Design review of the part shown in the three views and the two pictorial views. Dimensions are in mm from the part's minimum x, y and z. Give positions to 0.01 mm unless a question says otherwise; leave off trailing zeros. Loops run counter-clockwise (first coordinate to the right, second up) from the corner with the lowest first, then second, coordinate; pieces in that order, holes last.
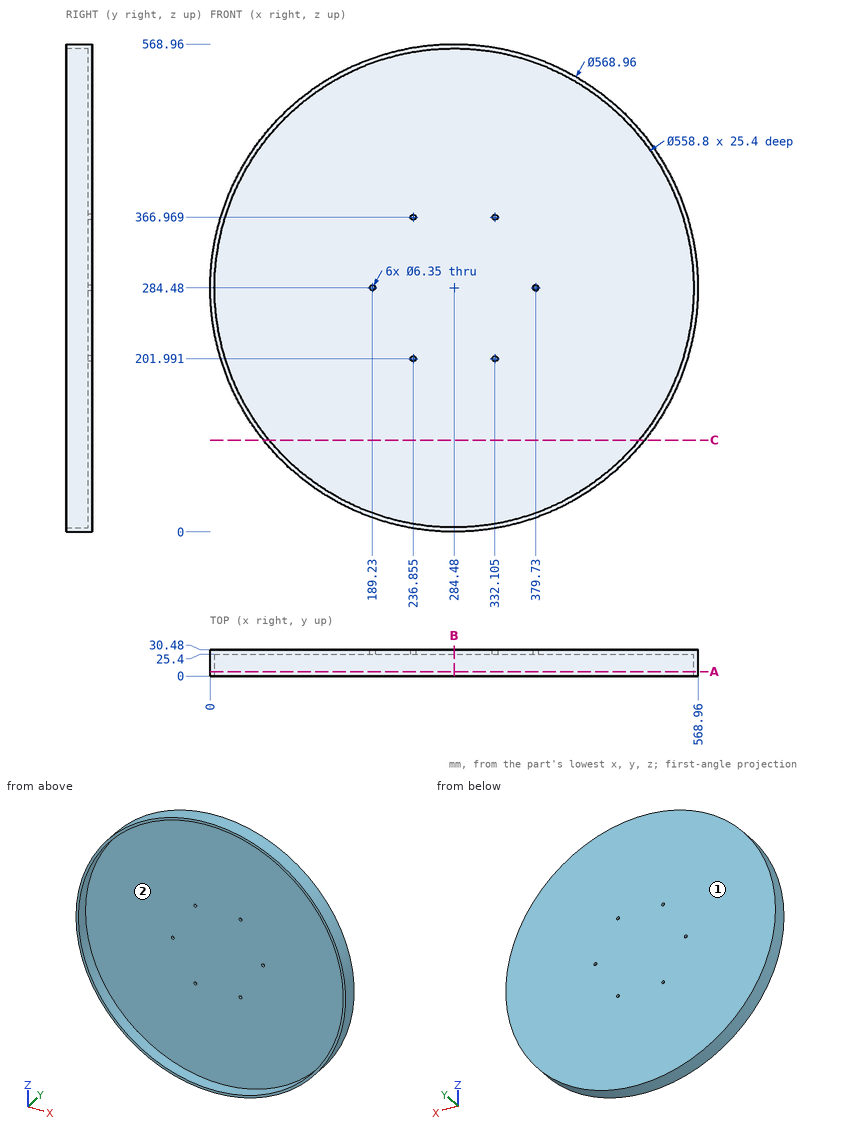
Q1. Mouldability with a two-part tool opening along X and no side actions: class the marked faces 1 and 2 as +X half, -X half, draft (parallel to the pull), parting line (faces both ways), or undercut.
Answers:
face 1: draft
face 2: undercut
Q2. For probe 1 along Z at (x, y) = (284, 12); probe 2 along Y at (x, z) = (367, 379); probe 3 along Z at (x, y) = (189.23, 27.1) (1 decimal), list the stretches that pass through material, from the lowest coordinate up.
Answers:
probe 1: z = 0 to 5.08, 563.88 to 568.96
probe 2: y = 25.4 to 30.48
probe 3: z = 16.4 to 281.3, 287.7 to 552.5
Q3. Consider section A-A on y = 5. Give the boundary of the cut face in (x, z), plus the area to 3 significant figures.
Answers:
outline: circle Ø568.96 at (284.48, 284.48); hole circle Ø558.8 at (284.48, 284.48)
area: 9,000 mm2
Q4. For pin 1 Ø5.5 at (x, z) = (236.86, 201.99) entering from -Y; pin 2 Ø3 at (y, z) = (15, 386) entering from -X; pin 3 Ø8 at (x, y) = (142.5, 21) entering from +Z; pin 4 Ø4 at (y, z) = (16.5, 422.5) entering from -X (3 decimals), all flat-tipped, find the tip position at first contact; note any pin that passes through.
Answers:
pin 1: passes through
pin 2: stops at x = 18.16
pin 3: stops at z = 533.26
pin 4: stops at x = 34.625
Q5. Consider section B-B on x = 284.48. Give the boundary of the cut face in (y, z).
Answers:
outline: (0, 0) - (30.48, 0) - (30.48, 568.96) - (0, 568.96) - (0, 563.88) - (25.4, 563.88) - (25.4, 5.08) - (0, 5.08) - close
Q6. Consider section C-C on z = 107. Give the boundary of the cut face in (x, y), plus the area to 3 significant figures.
Answers:
outline: (62.15, 0) - (68.69, 0) - (68.69, 25.4) - (500.27, 25.4) - (500.27, 0) - (506.81, 0) - (506.81, 30.48) - (62.15, 30.48) - close
area: 2,590 mm2
